Autodesk Inventor part; units mm, degrees
ref_plane "YZ Plane" through (0, 0, 0) normal (1, 0, 0) x (0, 1, 0)
ref_plane "XZ Plane" through (0, 0, 0) normal (0, 1, 0) x (-1, 0, 0)
ref_plane "XY Plane" through (0, 0, 0) normal (0, 0, 1) x (1, 0, 0)
sketch "スケッチ1" plane through (0, 0, 0) normal (0, 0, 1) x (1, 0, 0)
  circle A0 centre (0, 0) radius 34
  arc A1 (-4, 14.4568) -> (4, 14.4568) centre (0, 0) ccw
  line L0 (0, 15) -> (0, 11)
  line L1 (0, 15) -> (0, 18)
  line L2 (0, 18) -> (4, 18)
  line L3 (4, 18) -> (4, 14.4568)
  line L4 (4, 11) -> (0, 11)
  line L5 (0, 18) -> (-4, 18)
  line L6 (-4, 18) -> (-4, 14.4568)
  line L7 (-4, 11) -> (0, 11)
  point P0 (-4, 14.5)
  point P1 (4, 14.5)
  dimension "d0" = 68
  dimension "d1" = 30
  dimension "d2" = 4
  dimension "d3" = 3
  dimension "d4" = 4
extrude "押し出し1" add sketch "スケッチ1" along normal blind 40
properties part number "gear1"
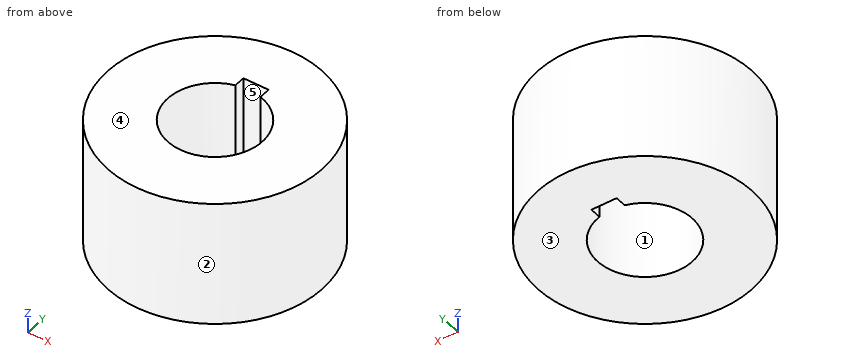
Build history of the part. All positions in model axes, mm. Face numbers are marked on the shaded views. A direction names the side the tool comes from. Coordinates: 2 decimals unless noted, no trailing zeros. Order: outer loops, then holes, each group sorted by start corner. A loop starts at its lowest first (then second) coordinate and runs counter-clockwise, first axis right, second up. Notation, with made-up numbers: M -10,44 L 36,44 A10 cw 36,60 Z; hole C 85.25,-11.75 d2. An arc over 180 degrees is marked long. One line per question, with ' | ' between items. Start each with the question number.
Q1. Two-plate mould, pull along Y, no slides. Class the marked faces 1, 2 and 3: +Y half, -Y half, draft (parallel to the pull), parting line (faces both ways), or undercut.
Q2. 3-axis set-ups, long thin cutter, end or side, ignore diameter. For the marked faces 4 and 5: which of +Z, -Z, +X, -X, +Y, -Y reach the whole face in a straight line?
Q3. Probe L1, parallel to Y at x = 0, z = 9.5; L2, parallel to X at y = -13, z = 10; L3, parallel to X at y = 0.5, z = 31. List the from-to ranges inside material, lowest first. Write a range as from..to.
Q4. Flat gauge pins, fed straight in: pin 1 Ø8 at (x, z) = (-23.5, 17) entering from -Y; pin 2 Ø1.8 at (y, z) = (16.5, 27) entering from -X; pin 3 Ø4 at (y, z) = (-11, 9) entering from +X. Where does each tip first touch, or does it go through?
Q5. Saw through at A-A (y = 0). List the corners of the cut face in (x, z), then the cut area to 3 significant figures.
Q6. Saw through at B-B (x = 0). List the corners of the cut face in (y, z).
Q7. Saw through at D-D (x = -30). List the corners of the cut face in (y, z), then the cut area to 3 significant figures.
Q8. Saw through at C-C (z = 16). List the corners of the cut face in (x, y).
Check values:
1) face 1: undercut | face 2: parting line | face 3: draft
2) face 4: +Z, +X, -X, +Y, -Y | face 5: +Z, -Z
3) L1: y = -34..-15, 18..34 | L2: x = -31.42..-7.48, 7.48..31.42 | L3: x = -34..-14.99, 14.99..34
4) pin 1: stops at y = -27.85 | pin 2: stops at x = -30.21 | pin 3: stops at x = 32.79
5) outline: M -34,0 L -15,0 L -15,40 L -34,40 Z; M 15,0 L 34,0 L 34,40 L 15,40 Z | area: 1,520 mm2
6) outline: M -34,0 L -15,0 L -15,40 L -34,40 Z; M 18,0 L 34,0 L 34,40 L 18,40 Z
7) outline: M -16,0 L 16,0 L 16,40 L -16,40 Z | area: 1,280 mm2
8) outline: C 0,0 d68; hole M -4,14.46 A15 ccw long 4,14.46 L 4,18 L -4,18 Z
